Work out the finished part from the listing and answer in its coordinate system (mm). A direction names the side the tool comes from. Round coordinates to 2 decimals unless told otherwise and drop trailing zeros. Loops run counter-clockwise (first coordinate to the right, second up) from the corner with the lowest first, then second, coordinate; pieces in that order, holes last.
Autodesk Inventor part; units mm, degrees
ref_plane "YZ Plane" through (0, 0, 0) normal (1, 0, 0) x (0, 1, 0)
ref_plane "XZ Plane" through (0, 0, 0) normal (0, 1, 0) x (-1, 0, 0)
ref_plane "XY Plane" through (0, 0, 0) normal (0, 0, 1) x (1, 0, 0)
sketch "Sketch14" plane through (0, 0, 0) normal (0, 0, 1) x (1, 0, 0)
  line L0 (0, 0) -> (-6.08, 0)
  line L1 (-6.08, 0) -> (0, 0)
  line L2 (0, 0) -> (6.08, 0)
  line L3 (-6.08, 0) -> (-6.08, 5)
  line L4 (-6.08, 0) -> (-1.08, 0) construction
  line L5 (-6.08, 5) -> (6.08, 5)
  line L6 (6.08, 5) -> (6.08, -5)
  line L7 (6.08, -5) -> (-6.08, -5)
  line L8 (-6.08, -5) -> (-6.08, 5)
  dimension "d66" = 6.08
  dimension "d67" = 6.08
  dimension "d68" = 5
  dimension "d69" = 90
  dimension "d70" = 12.16
  dimension "d71" = 10
extrude "Extrusion7" add sketch "Sketch14" along normal blind 2
sketch "Sketch15" plane through (0, 0, 2) normal (0, 0, 1) x (1, 0, 0)
  circle A0 centre (0, 0) radius 1.0665
hole "Hole4" at (0, 0, 2) direction (0, 0, -1) diameter 4.5 end through all
sketch "Sketch16" plane through (0, 0, 2) normal (0, 0, 1) x (1, 0, 0)
  line L0 (6.08, 5) -> (-6.08, 5)
  line L1 (0, 5) -> (10, 5)
  line L2 (10, 5) -> (-25.7, 5)
  line L3 (-25.7, 5) -> (-25.7, 37.05)
  line L4 (-25.7, 37.05) -> (10, 37.05)
  line L5 (10, 37.05) -> (10, 5)
  line L6 (-6.08, -5) -> (6.08, -5)
  line L7 (0, -5) -> (10, -5)
  line L8 (10, -5) -> (-25.7, -5)
  line L9 (-25.7, -5) -> (-25.7, -37.05)
  line L10 (-25.7, -37.05) -> (10, -37.05)
  line L11 (10, -37.05) -> (10, -5)
  line L12 (-25.7, 37.05) -> (-22.7, 37.05)
  line L13 (-22.7, 37.05) -> (-22.7, 34.05)
  line L14 (-22.7, 34.05) -> (-25.7, 34.05)
  line L15 (-25.7, 34.05) -> (-25.7, 37.05)
  line L16 (-22.7, 34.05) -> (7, 34.05)
  line L17 (7, 34.05) -> (7, 8)
  line L18 (7, 8) -> (-22.7, 8)
  line L19 (-22.7, 8) -> (-22.7, 34.05)
  line L20 (-25.7, -37.05) -> (-22.7, -37.05)
  line L21 (-22.7, -37.05) -> (-22.7, -34.05)
  line L22 (-22.7, -34.05) -> (-25.7, -34.05)
  line L23 (-25.7, -34.05) -> (-25.7, -37.05)
  line L24 (-22.7, -34.05) -> (7, -34.05)
  line L25 (7, -34.05) -> (7, -8)
  line L26 (7, -8) -> (-22.7, -8)
  line L27 (-22.7, -8) -> (-22.7, -34.05)
  line L28 (-25.7, -5) -> (10, -5)
  line L29 (10, -5) -> (10, -37.05)
  line L30 (10, -37.05) -> (-25.7, -37.05)
  line L31 (-25.7, -37.05) -> (-25.7, -5)
  point P0 (0, 0)
  dimension "d81" = 10
  dimension "d82" = 35.7
  dimension "d83" = 32.05
  dimension "d84" = 35.7
  dimension "d85" = 32.05
  dimension "d86" = 3
  dimension "d87" = 3
  dimension "d88" = 29.7
  dimension "d89" = 26.05
  dimension "d90" = 3
  dimension "d91" = 3
  dimension "d92" = 29.7
  dimension "d93" = 26.05
  dimension "d172" = 10
extrude "Extrusion8" add sketch "Sketch16" along normal blind 1.5 contours L16 L17 L18 L19 | L0 L2 L3 L14 L13 L4 L5 L1 | L13 L14 L3 L4 | L27 L26 L25 L24 | L6 L7 L11 L10 L21 L22 L9 L8 | L22 L21 L10 L9
hole "Hole5" at (-22.7, 34.05, 2) at (-22.7, 8, 2) at (7, 8, 2) at (7, 34.05, 2) at (7, -8, 2) at (7, -34.05, 2) at (-22.7, -34.05, 2) at (-22.7, -8, 2) direction (0, 0, 1) diameter 3.9 end through all
sketch "Sketch17" plane through (0, 0, 2) normal (0, 0, 1) x (1, 0, 0)
  circle A0 centre (0, 0) radius 2.25
  line L0 (6.08, -5) -> (6.08, 5)
  line L1 (6.08, 5) -> (-6.08, 5)
  line L2 (-6.08, 5) -> (-6.08, -5)
  line L3 (-6.08, -5) -> (6.08, -5)
extrude "Extrusion9" add sketch "Sketch17" along normal blind 4
sketch "Sketch18" plane through (6.08, -5, 0) normal (1, 0, 0) x (0, 0, -1)
  line L0 (0, 0) -> (0, 10)
  line L1 (0, 10) -> (-2, 10)
  line L2 (-3.5, 10) -> (-2, 10)
  line L3 (-3.5, 10) -> (-6, 10)
  line L4 (-6, 0) -> (-6, 10)
  line L5 (-3.5, 0) -> (-6, 0)
  line L6 (-2, 0) -> (-3.5, 0)
  line L7 (0, 0) -> (-2, 0)
  point P0 (0, 5)
extrude "Extrusion10" add sketch "Sketch18" along normal blind 30
sketch "Sketch19" plane through (36.08, -5, 0) normal (1, 0, 0) x (0, 0, -1)
  line L0 (-6, 10) -> (-6, 0)
  line L1 (-6, 0) -> (-16, 0)
  line L2 (-16, 0) -> (-16, 50)
  line L3 (-16, 50) -> (29, 50)
  line L4 (29, 50) -> (29, 25)
  line L5 (29, 25) -> (0, 10)
  line L6 (0, 10) -> (0, 0)
  line L7 (0, 10) -> (0, 0)
  line L8 (0, 0) -> (-6, 0)
  point P0 (0, 5)
  dimension "d107" = 10
  dimension "d108" = 50
  dimension "d109" = 90
  dimension "d110" = 45
  dimension "d111" = 90
  dimension "d112" = 25
extrude "Extrusion11" add sketch "Sketch19" along normal blind 2.5
sketch "Sketch21" plane through (38.58, -5, 0) normal (1, 0, 0) x (0, 0, -1)
  line L0 (-3.5, 10) -> (-6, 10)
  line L1 (0, 10) -> (0, 24.05)
  line L2 (0, 10) -> (14.05, 10) construction
  line L3 (0, 24.05) -> (6.713, 24.05)
  point P0 (0, 5)
  point P1 (3, 10)
  point P2 (-2, 10)
  dimension "d118" = 14.05
  dimension "d119" = 90
  dimension "d120" = 6.713
  dimension "d121" = 90
hole "Hole6" at (38.58, 19.05, -6.713) direction (-1, 0, 0) diameter 10 end through all
sketch "Sketch22" plane through (38.58, -5, 0) normal (1, 0, 0) x (0, 0, -1)
  circle A0 centre (6.713, 24.05) radius 5
  line L0 (6.713, 24.05) -> (6.713, 32.05)
  line L1 (6.713, 24.05) -> (14.713, 24.05) construction
  line L2 (6.713, 32.05) -> (24.213, 32.05)
  line L3 (24.213, 32.05) -> (-10.787, 32.05)
  point P0 (0, 5)
  dimension "d129" = 8
  dimension "d130" = 90
  dimension "d131" = 17.5
  dimension "d132" = 90
  dimension "d133" = 35
hole "Hole7" at (38.58, 27.05, 10.787) at (38.58, 27.05, -24.213) direction (-1, 0, 0) diameter 4.2 end through all
sketch "Sketch23" plane through (38.58, -5, 0) normal (1, 0, 0) x (0, 0, -1)
  line L0 (-3.5, 0) -> (-2, 0)
  line L1 (-2, 0) -> (-2, -9)
  line L2 (-2, 0) -> (7, 0) construction
  line L3 (-2, -9) -> (33, -9) construction
  line L4 (-2, -9) -> (33, -9)
  line L5 (-2, -9) -> (33, -9) construction
  line L6 (33, -9) -> (40.7782, -1.2218)
  line L7 (40.7782, -1.2218) -> (60.7782, -1.2218)
  line L8 (33, -9) -> (68, -9)
  line L9 (33, -9) -> (68, -9) construction
  line L10 (68, -9) -> (68, -1.2218)
  line L11 (68, -1.2218) -> (60.7782, -1.2218)
  line L12 (68, -9) -> (68, -29)
  line L13 (68, -9) -> (88, -9) construction
  line L14 (68, -29) -> (-2, -29)
  line L15 (-2, -29) -> (-2, -9)
  line L16 (33, -9) -> (44.45, -9)
  line L17 (44.45, -9) -> (44.45, -13.669)
  line L18 (44.45, -9) -> (49.119, -9) construction
  line L19 (44.45, -13.669) -> (44.45, -21.669)
  line L20 (44.45, -21.669) -> (61.95, -21.669)
  line L21 (61.95, -21.669) -> (26.95, -21.669)
  circle A0 centre (26.95, -21.669) radius 2.1
  circle A1 centre (61.95, -21.669) radius 2.1
  circle A2 centre (44.45, -13.669) radius 5
  point P0 (0, 5)
  dimension "d141" = 9
  dimension "d142" = 90
  dimension "d145" = 35
  dimension "d146" = 0
  dimension "d147" = 11
  dimension "d148" = 135
  dimension "d149" = 20
  dimension "d150" = 35
  dimension "d151" = 0
  dimension "d152" = 20
  dimension "d153" = 90
  dimension "d154" = 90
  dimension "d155" = 11.45
  dimension "d156" = 4.669
  dimension "d157" = 90
  dimension "d158" = 8
  dimension "d159" = 17.5
  dimension "d160" = 35
  dimension "d161" = 4.2
  dimension "d162" = 4.2
  dimension "d163" = 10
extrude "Extrusion13" add sketch "Sketch23" against normal blind 2 contours L4 L8 A2 L12 L14 L15 | L6 L7 L11 L10 L8 A2
sketch "Sketch24" plane through (38.58, -5, 0) normal (1, 0, 0) x (0, 0, -1)
  line L0 (-16, 50) -> (-16, 0)
  line L1 (-16, 0) -> (-16, -29)
  line L2 (68, -29) -> (-2, -29)
  line L3 (-16, -29) -> (-2, -29)
  line L4 (0, 0) -> (-2, 0)
  line L5 (-2, -29) -> (-2, 0)
  line L6 (-16, 0) -> (0, 0)
  line L7 (-2, 0) -> (-16, 0)
  point P0 (0, 5)
  point P1 (3, 0)
extrude "Extrusion14" add sketch "Sketch24" against normal blind 2
sketch "Sketch25" plane through (36.58, -5, 0) normal (-1, 0, 0) x (0, 0, 1)
  line L0 (2, -9) -> (-33, -9)
  line L1 (-33, -9) -> (2, -9)
  line L2 (2, -9) -> (2, -11)
  line L3 (2, -11) -> (-33, -11)
  line L4 (-33, -11) -> (-33, -9)
  line L5 (2, -11) -> (6, -11)
  line L6 (6, -11) -> (6, 0)
  line L7 (6, 0) -> (2, 0)
  line L8 (2, 0) -> (2, -11)
  point P0 (0, 5)
  point P1 (2, -9)
  dimension "d168" = 35
  dimension "d169" = 2
extrude "Extrusion15" add sketch "Sketch25" along normal blind 10
sketch "Sketch26" plane through (38.58, -5, 0) normal (1, 0, 0) x (0, 0, -1)
  line L0 (29, 50) -> (-16, 50)
  line L1 (-16, 50) -> (29, 50)
  line L2 (29, 50) -> (29, 10)
  line L3 (29, 10) -> (-16, 10)
  line L4 (-16, 10) -> (-16, 50)
  dimension "d173" = 40
extrude "Extrusion16" cut sketch "Sketch26" against normal up to surface (64.28 mm away)
sketch "Sketch27" plane through (10, -37.05, 2) normal (1, 0, 0) x (0, 0, -1)
  line L0 (-1.5, 0) -> (-4, 0)
  line L1 (0, 32.05) -> (-4, 32.05)
  line L2 (-4, 0) -> (-4, 32.05)
  line L3 (0, 32.05) -> (2, 32.05)
  line L4 (-4, 32.05) -> (2, 32.05)
  line L5 (2, 32.05) -> (2, 0)
  line L6 (2, 0) -> (-1.5, 0)
  point P0 (2, 37.05)
extrude "Extrusion17" add sketch "Sketch27" along normal up to surface (26.58 mm away)
sketch "Sketch28" plane through (36.08, -5, 16) normal (0, 0, 1) x (1, 0, 0)
  line L0 (2.5, 0) -> (2.5, 10)
  line L1 (-26.08, -32.05) -> (-26.08, 0)
  line L2 (2.5, 10) -> (-26.08, 10)
  line L3 (-26.08, 10) -> (-26.08, -9.2291)
  line L4 (-26.08, -9.2291) -> (2.5, -9.2291)
  line L5 (2.5, -9.2291) -> (2.5, 10)
  point P0 (-36.08, 5)
extrude "Extrusion18" cut sketch "Sketch28" against normal up to surface (49 mm away)
sketch "Sketch29" plane through (0, 0, 6) normal (0, 0, 1) x (1, 0, 0)
  line L0 (-6.08, 5) -> (10, 5)
  line L1 (-6.08, -5) -> (6.08, -5)
  line L2 (6.08, -5) -> (6.08, 5)
  line L3 (6.08, 5) -> (-6.08, 5)
  line L4 (-6.08, 5) -> (-6.08, -5)
  line L5 (10, 5) -> (6.08, 5)
  line L6 (6.08, 5) -> (6.08, -5)
  line L7 (6.08, -5) -> (10, -5)
  line L8 (10, -5) -> (10, 5)
  point P0 (0, 0)
  dimension "d180" = 12.16
extrude "Extrusion19" cut sketch "Sketch29" against normal blind 10 contours L0 L8 L7 L2
sketch "Sketch30" plane through (36.58, -14.2291, 16) normal (0, 1, 0) x (1, 0, 0)
  line L0 (-10, 49) -> (-10, 16)
  line L1 (0, 84) -> (0, 16)
  line L2 (-10, 49) -> (0, 49)
  line L3 (0, 49) -> (0, 33)
  line L4 (0, 33) -> (-10, 33)
  line L5 (-10, 33) -> (-10, 49)
  point P0 (-36.58, 16)
  dimension "d183" = 16
extrude "Extrusion20" cut sketch "Sketch30" against normal blind 10
sketch "Sketch31" plane through (0, 0, 0) normal (0, 0, -1) x (-1, 0, 0)
  line L0 (6.08, 5) -> (6.08, -5)
  line L1 (-6.08, -5) -> (6.08, -5)
  line L2 (6.08, 5) -> (5.08, 5)
  line L3 (5.08, 5) -> (5.08, -5)
  line L4 (5.08, -5) -> (6.08, -5)
  line L5 (6.08, -5) -> (6.08, 5)
  point P0 (0, 0)
  dimension "d186" = 1
extrude "Extrusion21" add sketch "Sketch31" along normal blind 5
properties part number "Shelf_half_left"
1. Find section A-A (z = -44.45). Write down the section's boundary in (x, y).
Answer key:
outline: (36.58, -34) - (38.58, -34) - (38.58, -23.67) - (36.58, -23.67) - close; (36.58, -13.67) - (38.58, -13.67) - (38.58, -6.22) - (36.58, -6.22) - close
2. Find section B-B (x = -22.7). Write down the section's boundary in (y, z), then the cut area to 3 significant figures.
Answer key:
outline: (-37.05, 2) - (-36, 2) - (-36, 3.5) - (-37.05, 3.5) - close; (-32.1, 2) - (-9.95, 2) - (-9.95, 3.5) - (-32.1, 3.5) - close; (-6.05, 2) - (-5, 2) - (-5, 3.5) - (-6.05, 3.5) - close
area: 36.4 mm2
3. Consider probe 1 along Y at (x, z) = (7, 2.4); probe 2 along X at (y, z) = (-34.05, 2.6); probe 3 along X at (y, z) = (-25, -41). Determine where each line is inside the solid, lowest interval first.
Answer key:
probe 1: y = -37.05 to -36, -32.1 to -9.95, -6.05 to -5
probe 2: x = -25.7 to -24.65, -20.75 to 5.05, 8.95 to 36.58
probe 3: x = 36.58 to 38.58
4. Find section D-D (z = -61.95). Write down the section's boundary in (x, y), then the cut area to 3 significant figures.
Answer key:
outline: (36.58, -34) - (38.58, -34) - (38.58, -28.77) - (36.58, -28.77) - close; (36.58, -24.57) - (38.58, -24.57) - (38.58, -6.22) - (36.58, -6.22) - close
area: 47.2 mm2
5. Which of the six approach directions +Z, -Z, +X, -X, +Y, -Y give full straight-line access (tool end or side, diameter ignored) to faces 4 (the face through (3, 0, 0)), 5 (the face through (36.58, -24, 11)), 6 (the face through (30, -14.229, -3))?
Answer key:
face 4: -Z, +X, +Y, -Y
face 5: +Z, -X, +Y, -Y
face 6: +Z, +X, +Y
6. Determine the mould class of faces 1 (the face through (-20.97, -33.15, 2.76)), 2 (the face through (26.58, -15, -9)), 3 (the face through (38, -20, -68)) for opening direction X: +X half, -X half, draft (parallel to the pull), parting line (faces both ways), or undercut.
Answer key:
face 1: undercut
face 2: -X half
face 3: draft
7. Given pin 1 (3 mm diameter, centred on x = 29.5, z = -5.5, fed in from -Y); pin 2 (1.5 mm diameter, centred on y = -2.5, z = -2.5, fed in from +X); pin 3 (1.4 mm diameter, centred on x = 30, y = -15, fed in from -Z), each flat-ended and moving along its own axis, determine where each tip first touches the part or whether it passes through.
Answer key:
pin 1: stops at y = -16
pin 2: stops at x = -5.08
pin 3: stops at z = -17
8. Find section C-C (y = -8). Write down the section's boundary in (x, z).
Answer key:
outline: (-25.7, 2) - (-24.65, 2) - (-24.65, 3.5) - (-25.7, 3.5) - close; (-20.75, 2) - (5.05, 2) - (5.05, 3.5) - (-20.75, 3.5) - close; (8.95, 2) - (10, 2) - (10, 3.5) - (8.95, 3.5) - close; (36.58, -68) - (38.58, -68) - (38.58, -39) - (36.58, -39) - close
